from build123d import *

# Parameters (mm, degrees)
F1_DEPTH = 15
F2_W     = 21
F2_H     = 38.66523
F3_DEPTH = 2


with BuildPart() as f1:
    # F0 (on Front) → F1 (new body)
    with BuildSketch(Plane.XZ):
        with BuildLine():
            Line((-10.5, 19.332615), (-10.5, -19.332615))
            ThreePointArc((-10.5, -19.332615), (0, -22), (10.5, -19.332615))
            Line((10.5, -19.332615), (10.5, 19.332615))
            ThreePointArc((10.5, 19.332615), (0, 22), (-10.5, 19.332615))
        make_face()
        with BuildLine():
            ThreePointArc((-5.500001, 16.085709), (0, 17.000001), (5.500001, 16.085709))
            Line((5.500001, 16.085709), (5.500001, -16.085709))
            ThreePointArc((5.500001, -16.085709), (0, -17.000001), (-5.500001, -16.085709))
            Line((-5.500001, -16.085709), (-5.500001, 16.085709))
        make_face(mode=Mode.SUBTRACT)
    extrude(amount=F1_DEPTH)

    # F2 (on face) → F3 (join)
    with BuildSketch(Plane.XZ.offset(15)):
        with BuildLine():
            ThreePointArc((10.5, 19.332615), (0, 22), (-10.5, 19.332615))
            Line((-10.5, 19.332615), (10.5, 19.332615))
        make_face()
        Rectangle(F2_W, F2_H)
        with BuildLine():
            Line((10.5, -19.332615), (-10.5, -19.332615))
            ThreePointArc((-10.5, -19.332615), (0, -22), (10.5, -19.332615))
        make_face()
    extrude(amount=F3_DEPTH)


solid = f1.part
The model under review builds one solid part; all positions refer to its coordinate system, in mm. A direction names the side the tool comes from. Round coordinates to 2 decimals unless told otherwise and drop trailing zeros. Order: outer loops, then holes, each group sorted by start corner. A loop starts at its lowest first (then second) coordinate and runs counter-clockwise, first axis right, second up. Notation, with made-up numbers: (4.5, -30.5) -> (44.5, -30.5) arc R35 ccw to (44.5, 2.5) -> close; hole circle Ø11 at (24.5, 6). An arc over 180 degrees is marked (long way). Return JSON: item names as keys, results as strings.
1. For faces 5 (the face through (0, -7, 17)), 6 (the face through (0, -8, 22)), list the 3-axis set-ups (+Z, -Z, +X, -X, +Y, -Y) from which the entire face can be reached by the end or side of a thin tool; tool diameter is ignored.
Answer block:
{"face 5": "+Y", "face 6": "+Z, +Y, -Y"}
2. Take a section at A-A (z = 3.5). Write out the cut boundary in (x, y).
Answer block:
{"outline": "(-10.5, -17) -> (10.5, -17) -> (10.5, 0) -> (5.5, 0) -> (5.5, -15) -> (-5.5, -15) -> (-5.5, 0) -> (-10.5, 0) -> close"}
3. Insertion check: P1, Ø5.5, axis at x = -1.5, z = -4.5, coming from the +Y side. The pin has a flat end and moves straight along its axis. Give the tip position at first contact, or say it passes through.
Answer block:
{"P1": "stops at y = -15"}
4. Take a section at B-B (y = -12.25). Write out the cut boundary in (x, z), then the cut area to 3 significant figures.
Answer block:
{"outline": "(-10.5, -19.33) arc R22 ccw to (10.5, -19.33) -> (10.5, 19.33) arc R22 ccw to (-10.5, 19.33) -> close; hole (-5.5, -16.09) arc R17 ccw to (5.5, -16.09) -> (5.5, 16.09) arc R17 ccw to (-5.5, 16.09) -> close", "area": "520 mm²"}
5. For L1, parallel to X at y = -12.25, z = -2; L2, parallel to Z at x = 0.25, y = -8; L3, parallel to Y at x = -0.5, z = -16, list the stretches that pass through material, from the lowest coordinate up. Write a range as [from, to].
Answer block:
{"L1": "x = [-10.5, -5.5], [5.5, 10.5]", "L2": "z = [-22, -17], [17, 22]", "L3": "y = [-17, -15]"}
6. The part is to be moulded in two halves that separate along X. For faces 1 (the face through (-5.5, -7, 0)), 2 (the face through (10.5, -8, 0)), 3 (the face through (0, -17, 0)), 4 (the face through (-10.5, -8, 0)), say which applies: +X half, -X half, draft (parallel to the pull), parting line (faces both ways), or undercut.
Answer block:
{"face 1": "undercut", "face 2": "+X half", "face 3": "draft", "face 4": "-X half"}
7. Take a section at C-C (x = -4). Write out the cut boundary in (y, z), then the cut area to 3 significant figures.
Answer block:
{"outline": "(-17, -21.63) -> (0, -21.63) -> (0, -16.52) -> (-15, -16.52) -> (-15, 16.52) -> (0, 16.52) -> (0, 21.63) -> (-17, 21.63) -> close", "area": "240 mm²"}
